The model under review builds one solid part; all positions refer to its coordinate system, in mm. A direction names the side the tool comes from. Coordinates: 2 decimals unless noted, no trailing zeros. Order: outer loops, then holes, each group sorted by start corner. A loop starts at its lowest first (then second) coordinate and runs counter-clockwise, first axis right, second up. Notation, with made-up numbers: M 10,88.25 L 67,88.25 A28 cw 67,126.25 Z; hole C -1,11.5 d7. An arc over 180 degrees is marked long. Write each question's results on one line, items separated by ' | '.
from build123d import *

# Parameters (mm, degrees)
SKETCH1_W                  = 487
SKETCH1_H                  = 270
BOSS_EXTRUDE1_DEPTH        = 1.5875
SKETCH2_R                  = 135
SKETCH2_R_2                = 115
CUT_EXTRUDE1_DEPTH         = 557.840659575
SKETCHED_BEND2_DEPTH       = 270
SKETCHED_BEND2_2_DEPTH     = 270
SKETCHED_START             = -1
SKETCHED_BEND2_3_OUTLINE_W = 1.5875
SKETCHED_BEND2_3_OUTLINE_H = 270
SKETCHED_BEND2_3_DEPTH     = 161
SKETCHED_START_2           = 326
SKETCHED_BEND2_4_DEPTH     = 1.5875
SKETCHED_START_3           = 158.4125
SKETCHED_BEND2_5_DEPTH     = 11.5875
SKETCHED_BEND2_6_DEPTH     = 270


with BuildPart() as part:
    # Sketch1 → Boss-Extrude1 (new body)
    with BuildSketch(Plane(origin=(0, 0, 0), x_dir=(1, 0, 0), z_dir=(0, 1, 0))):
        with Locations((243.5, -135)):
            Rectangle(SKETCH1_W, SKETCH1_H)
    extrude(amount=BOSS_EXTRUDE1_DEPTH)

    # Sketch2 → Cut-Extrude1 (cut, through all)
    with BuildSketch(Plane(origin=(0, 1.5875, 0), x_dir=(1, 0, 0), z_dir=(0, 1, 0))):
        with Locations((0, -135)):
            Circle(SKETCH2_R)
        with Locations((487, -135)):
            Circle(SKETCH2_R_2)
    extrude(amount=-CUT_EXTRUDE1_DEPTH, mode=Mode.SUBTRACT)

    # Sketched Bend2: read off the stored shape, not the designer's step
    # Sketched Bend2 outline → Sketched Bend2 (cut)
    with BuildSketch(Plane.XY):
        with BuildLine():
            ThreePointArc((321.854071767, 1.5875), (319.032750917, 0.403914791), (316, 0))
            Line((316, 0), (487, 0))
            Line((487, 0), (487, 1.5875))
            Line((487, 1.5875), (321.854071767, 1.5875))
        make_face()
    extrude(amount=SKETCHED_BEND2_DEPTH, mode=Mode.SUBTRACT)

    # Sketched Bend2 2 outline → Sketched Bend2 2 (add)
    with BuildSketch(Plane.XY):
        with BuildLine():
            ThreePointArc((326, 11.5875), (323.071067812, 4.516432188), (316, 1.5875))
            Line((316, 1.5875), (321.854071767, 1.5875))
            ThreePointArc((321.854071767, 1.5875), (326.052467678, 5.8239898), (327.5875, 11.5875))
            Line((327.5875, 11.5875), (327.5875, 165.632717148))
            Line((327.5875, 165.632717148), (326, 165.632717148))
            Line((326, 165.632717148), (326, 11.5875))
        make_face()
    extrude(amount=SKETCHED_BEND2_2_DEPTH)

    # Sketched Bend2 3 outline → Sketched Bend2 3 (cut)
    with BuildSketch(Plane.YZ.offset(SKETCHED_START)):
        with Locations((0.79375, 135)):
            Rectangle(SKETCHED_BEND2_3_OUTLINE_W, SKETCHED_BEND2_3_OUTLINE_H)
    extrude(amount=SKETCHED_BEND2_3_DEPTH, mode=Mode.SUBTRACT)

    # Sketched Bend2 4 outline → Sketched Bend2 4 (cut)
    with BuildSketch(Plane.YZ.offset(SKETCHED_START_2)):
        with BuildLine():
            ThreePointArc((165.632717148, 250), (50.632717148, 135), (165.632717148, 20))
            Line((165.632717148, 20), (165.632717148, 250))
        make_face()
    extrude(amount=SKETCHED_BEND2_4_DEPTH, mode=Mode.SUBTRACT)

    # Sketched Bend2 5 outline → Sketched Bend2 5 (add)
    with BuildSketch(Plane.YZ.offset(SKETCHED_START_3)):
        with BuildLine():
            Line((164.632717148, 270), (1.5875, 270))
            Line((1.5875, 270), (1.5875, 0))
            Line((1.5875, 0), (164.632717148, 0))
            ThreePointArc((164.632717148, 0), (29.632717148, 135), (164.632717148, 270))
        make_face()
    extrude(amount=SKETCHED_BEND2_5_DEPTH)

    # Sketched Bend2 6 outline → Sketched Bend2 6 (cut)
    with BuildSketch(Plane.XY):
        with BuildLine():
            Line((160, 167), (160, 11.5875))
            ThreePointArc((160, 11.5875), (162.928932188, 4.516432188), (170, 1.5875))
            Line((170, 1.5875), (170, 167))
            Line((170, 167), (160, 167))
        make_face()
        with BuildLine():
            Line((329, -2), (329, 0))
            Line((329, 0), (170, 0))
            ThreePointArc((170, 0), (161.806400173, 3.393900173), (158.4125, 11.5875))
            Line((158.4125, 11.5875), (158.4125, 1.5875))
            Line((158.4125, 1.5875), (160, 1.5875))
            Line((160, 1.5875), (160, -2))
            Line((160, -2), (329, -2))
        make_face()
    extrude(amount=SKETCHED_BEND2_6_DEPTH, mode=Mode.SUBTRACT)


solid = part.part
1) Take a section at D-D on y = 69. State the section outline as (x, z) points.
Solutions:
outline: M 158.41,0 L 160,0 L 160,39.71 L 158.41,39.71 Z; M 158.41,230.29 L 160,230.29 L 160,270 L 158.41,270 Z; M 326,0 L 327.59,0 L 327.59,72.65 L 326,72.65 Z; M 326,197.35 L 327.59,197.35 L 327.59,270 L 326,270 Z
2) Take a section at B-B on z = 135. State the section outline as (x, y) points (1 decimal), plus the area to 3 significant figures.
Solutions:
outline: M 158.4,11.6 A11.6 ccw 170,0 L 316,0 A11.6 ccw 327.6,11.6 L 327.6,50.6 L 326,50.6 L 326,11.6 A10 cw 316,1.6 L 170,1.6 A10 cw 160,11.6 L 160,29.6 L 158.4,29.6 Z | area: 376 mm2
3) Take a section at C-C on y = 127. State the section outline as (x, z) points, plus the area to 3 significant figures.
Solutions:
outline: M 158.41,0 L 160,0 L 160,5.35 L 158.41,5.35 Z; M 158.41,264.65 L 160,264.65 L 160,270 L 158.41,270 Z; M 326,0 L 327.59,0 L 327.59,26.68 L 326,26.68 Z; M 326,243.32 L 327.59,243.32 L 327.59,270 L 326,270 Z | area: 102 mm2
4) For pin 1 (5 mm diameter, centred on x = 279.5, z = 114.5, fed in from +Y), flat-tipped, find the tip position at first contact; note if it passes through.
Solutions:
pin 1: y = 1.59
5) For faces 4 (the flat face through (158.412, 25, 136)), 5 (the flat face through (242, 1.588, 133)), list the 3-axis set-ups (+Z, -Z, +X, -X, +Y, -Y) from which the entire face can be reached by the end or side of a thin tool; tool diameter is ignored.
Solutions:
face 4: +Z, -Z, -X, +Y, -Y | face 5: +Z, -Z, +Y
6) The part is to be moulded in two halves that separate along Z. For faces 1 (the cylindrical face through (159.195, 29.665, 132.031)), 2 (the cylindrical face through (326.78, 50.66, 137.53)), 3 (the flat face through (326, 38, 133)), say which applies: pulls with the +Z half, pulls with the -Z half, needs draft (parallel to the pull), parting line crosses it, or undercut.
Solutions:
face 1: undercut | face 2: undercut | face 3: needs draft
7) Take a section at A-A on y = 20.5. State the section outline as (x, z) points, plus the area to 3 significant figures.
Solutions:
outline: M 158.41,0 L 160,0 L 160,270 L 158.41,270 Z; M 326,0 L 327.59,0 L 327.59,270 L 326,270 Z | area: 857 mm2
8) To check wall thickness, follow line 1 along X through (y, z) = (22.5, 120.5); line 2 along Y through (x, z) = (298, 126); line 3 along X through (y, z) = (55, 200). State the ranges of each line that lie inside material, in increasing order.
Solutions:
line 1: 158.41 to 160, 326 to 327.59 | line 2: 0 to 1.59 | line 3: 326 to 327.59
